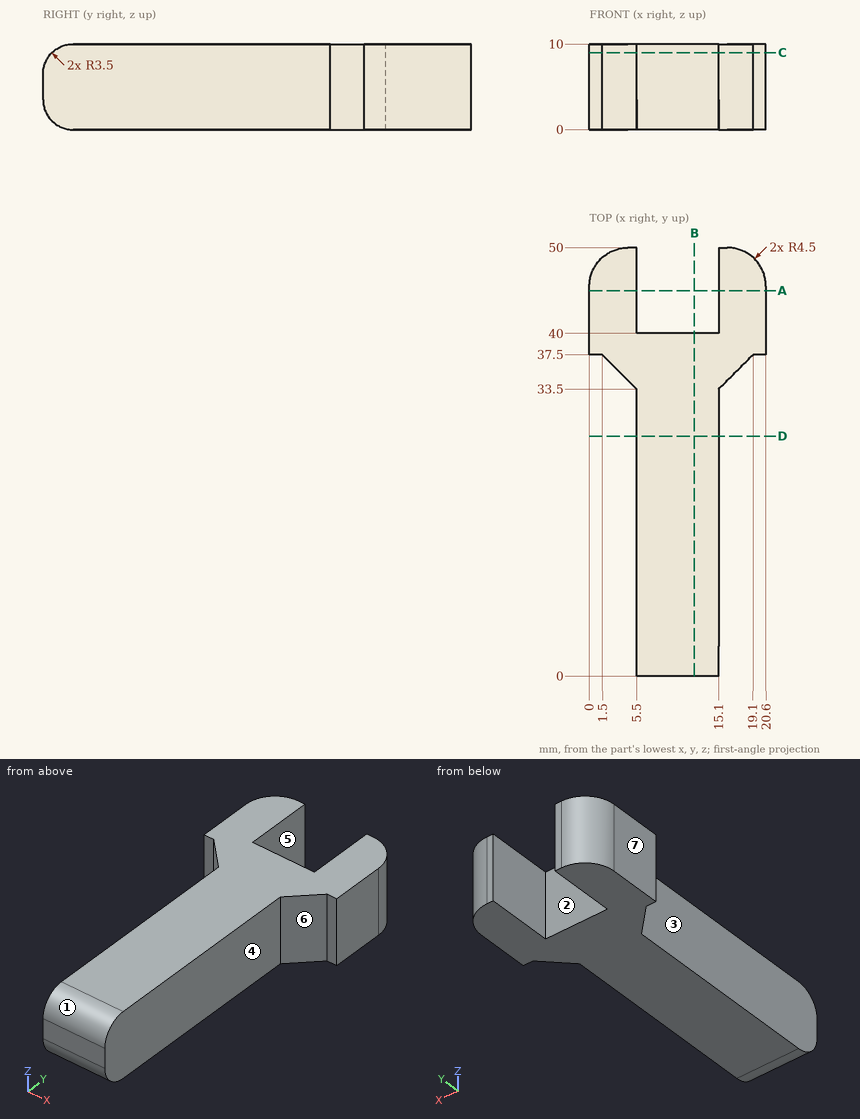
For this review, use the dimensioned drawing (mm, ordinates from the lowest corner) and the shaded views. A direction names the side the tool comes from. Round coordinates to 2 decimals unless told otherwise and drop trailing zeros. Write each loop counter-clockwise with the first axis right and the second up, starting at its lowest first coordinate (ties: lowest second). Pieces come first, ordered by that corner, then holes. Notation, with made-up numbers: (17, 30.5) -> (60, 30.5) arc R30 ccw to (60, 58.5) -> close; hole circle Ø6 at (69, -18). An arc over 180 degrees is marked (long way). One line per item, written item: value. Start each with the question number.
Q1. Add section B-B (x = 12.25). Give the boundary of the cut face in (y, z), then the cut area to 3 significant figures.
Q2. Add section C-C (z = 9). Give the boundary of the cut face in (x, y).
Q3. The part is to be moulded in two halves that separate along X. For the marked faces 5, 6 and 7, say which applies: pulls with the +X half, pulls with the -X half, needs draft (parallel to the pull), parting line crosses it, or undercut.
Q4. Add section D-D (y = 28). Give the boundary of the cut face in (x, z).
Q5. Tool access review of the marked faces 1, 2, 3 and 4: name each direction out of +Z, -Z, +X, -X, +Y, -Y from which nothing blocks a thin tool from reaching the whole face with its end or side.
Q6. Add section A-A (y = 45). Give the boundary of the cut face in (x, z).
Q7. To check wall thickness, follow probe 1 along X at (y, z) = (16.5, 6.5); probe 2 along Y at (x, z) = (14.25, 5.5); probe 3 along Y at (x, z) = (7.75, 2.5). State the ranges of each line that lie inside material, in increasing order.
Q8. Insertion check: P1, Ø5, axis at x = 8.5, z = 3, coming from the +Y side; P2, Ø5, axis at y = 13, z = 6, coming from the +X side; P3, Ø1.5, axis at y = 16, z = 5.5, coming from the -X side. Each pin has a flat end and moves straight along its axis. Give the tip position at first contact, or say it passes through.
Response:
1. outline: (0, 3.5) arc R3.5 ccw to (3.5, 0) -> (40, 0) -> (40, 10) -> (3.5, 10) arc R3.5 ccw to (0, 6.5) -> close
1. area: 395 mm^2
2. outline: (0, 37.5) -> (1.5, 37.5) -> (5.5, 33.5) -> (5.5, 1.05) -> (15.1, 1.05) -> (15.1, 33.5) -> (19.1, 37.5) -> (20.6, 37.5) -> (20.6, 45.5) arc R4.5 ccw to (16.1, 50) -> (15.1, 50) -> (15.1, 40) -> (5.5, 40) -> (5.5, 50) -> (4.5, 50) arc R4.5 ccw to (0, 45.5) -> close
3. face 5: undercut
3. face 6: pulls with the +X half
3. face 7: pulls with the -X half
4. outline: (5.5, 0) -> (15.1, 0) -> (15.1, 10) -> (5.5, 10) -> close
5. face 1: +Z, +X, -X, -Y
5. face 2: +Z, -Z, +Y
5. face 3: +Z, -Z, -X, -Y
5. face 4: +Z, -Z, +X, -Y
6. outline: (0, 0) -> (5.5, 0) -> (5.5, 10) -> (0, 10) -> close; (15.1, 0) -> (20.6, 0) -> (20.6, 10) -> (15.1, 10) -> close
7. probe 1: x = 5.5 to 15.1
7. probe 2: y = 0 to 40
7. probe 3: y = 0.15 to 40
8. P1: stops at y = 40
8. P2: stops at x = 15.1
8. P3: stops at x = 5.5
